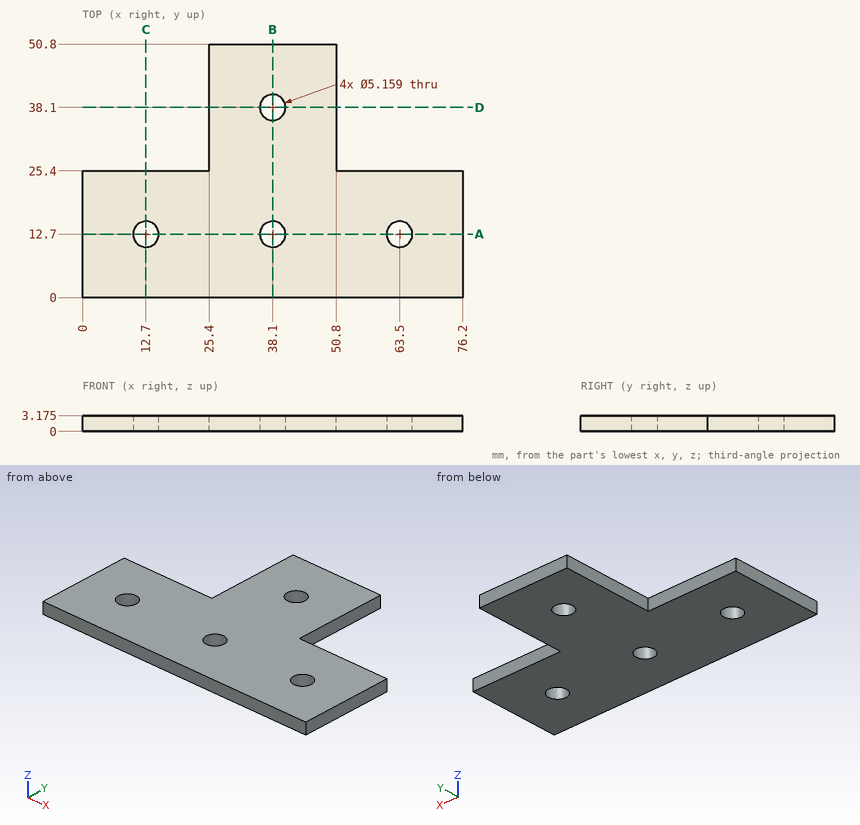
Part print with two shaded views. Sizes in mm from the minimum x, y, z corner. Coordinates: 2 decimals unless noted, no trailing zeros. Write each loop counter-clockwise with the first axis right and the second up, starting at its lowest first coordinate (ties: lowest second). Pieces come first, ordered by that corner, then holes. Notation, with made-up numbers: (87, 67) - (117, 67) arc R16 ccw to (117, 79) - close; hole circle Ø11 at (51, -16). An arc over 180 degrees is marked (long way). Use a Markdown table: item, result. Add a question column.
Item 1: Band-saw the part on A-A, the plane y = 12.7. Write the cut outline in (x, z) (1 decimal).
Item 2: Band-saw the part on C-C, the plane x = 12.7. Write the cut outline in (y, z) (1 decimal).
Item 3: Band-saw the part on B-B, the plane x = 38.1. Write the cut outline in (y, z) (1 decimal).
Item 4: Drill centre lines: line 1 along Y through (x, z) = (63.5, 1.15); line 2 along Y through (x, z) = (38.1, 1); line 3 along Y through (x, z) = (22, 2.3). Where is each one in solid material? Low to high.
Item 5: Drop flat-ended pins along their axis: pin 1 (8 mm diameter, centred on x = 68.5, y = 28, fed in from -Z); pin 2 (1.6 mm diameter, centred on y = 43, z = 1, fed in from +X); pin 3 (1.6 mm diameter, centred on x = 69, z = 2, fed in from +Y). Give the stop position or say it passes through.
Item 6: Band-saw the part on D-D, the plane y = 38.1. Write the cut outline in (x, z) (1 decimal).
A:
| question | item | result |
|---|---|---|
| 1 | outline | (0, 0) - (10.1, 0) - (10.1, 3.2) - (0, 3.2) - close; (15.3, 0) - (35.5, 0) - (35.5, 3.2) - (15.3, 3.2) - close; (40.7, 0) - (60.9, 0) - (60.9, 3.2) - (40.7, 3.2) - close; (66.1, 0) - (76.2, 0) - (76.2, 3.2) - (66.1, 3.2) - close |
| 2 | outline | (0, 0) - (10.1, 0) - (10.1, 3.2) - (0, 3.2) - close; (15.3, 0) - (25.4, 0) - (25.4, 3.2) - (15.3, 3.2) - close |
| 3 | outline | (0, 0) - (10.1, 0) - (10.1, 3.2) - (0, 3.2) - close; (15.3, 0) - (35.5, 0) - (35.5, 3.2) - (15.3, 3.2) - close; (40.7, 0) - (50.8, 0) - (50.8, 3.2) - (40.7, 3.2) - close |
| 4 | line 1 | y = 0 to 10.12, 15.28 to 25.4 |
| 4 | line 2 | y = 0 to 10.12, 15.28 to 35.52, 40.68 to 50.8 |
| 4 | line 3 | y = 0 to 25.4 |
| 5 | pin 1 | stops at z = 0 |
| 5 | pin 2 | stops at x = 50.8 |
| 5 | pin 3 | stops at y = 25.4 |
| 6 | outline | (25.4, 0) - (35.5, 0) - (35.5, 3.2) - (25.4, 3.2) - close; (40.7, 0) - (50.8, 0) - (50.8, 3.2) - (40.7, 3.2) - close |
